```python
from build123d import *

# Parameters (mm, degrees)
ESQUISSE1_R             = 53.5
ESQUISSE1_R_2           = 1
ESQUISSE1_R_3           = 3
BOSS_EXTRU_1_DEPTH      = 1.6
ENL_V_MAT_EXTRU_1_DEPTH = 76.677341391


with BuildPart() as part:
    # Esquisse1 → Boss.-Extru.1 (new body)
    with BuildSketch(Plane.XY):
        Circle(ESQUISSE1_R)
        with Locations((35, 0)):
            Circle(ESQUISSE1_R_2, mode=Mode.SUBTRACT)
        with Locations((17.5, -30.310889132)):
            Circle(ESQUISSE1_R_2, mode=Mode.SUBTRACT)
        with Locations((-17.5, -30.310889132)):
            Circle(ESQUISSE1_R_2, mode=Mode.SUBTRACT)
        with Locations((-35, 0)):
            Circle(ESQUISSE1_R_2, mode=Mode.SUBTRACT)
        with Locations((-17.5, 30.310889132)):
            Circle(ESQUISSE1_R_2, mode=Mode.SUBTRACT)
        with Locations((17.5, 30.310889132)):
            Circle(ESQUISSE1_R_2, mode=Mode.SUBTRACT)
        with Locations((0, -15)):
            Circle(ESQUISSE1_R_3, mode=Mode.SUBTRACT)
        with Locations((12.990381057, -7.5)):
            Circle(ESQUISSE1_R_3, mode=Mode.SUBTRACT)
        with Locations((12.990381057, 7.5)):
            Circle(ESQUISSE1_R_3, mode=Mode.SUBTRACT)
        with Locations((0, 15)):
            Circle(ESQUISSE1_R_3, mode=Mode.SUBTRACT)
        with Locations((-12.990381057, 7.5)):
            Circle(ESQUISSE1_R_3, mode=Mode.SUBTRACT)
    extrude(amount=BOSS_EXTRU_1_DEPTH)

    # Esquisse2 → Enlèv. mat.-Extru.1 (cut, through all)
    with BuildSketch(Plane.XY.offset(1.6)):
        with BuildLine():
            Line((-37.206596087, 38.4437148), (14.689935589, -51.4437148))
            ThreePointArc((14.689935589, -51.4437148), (-46.332359102, -26.75), (-37.206596087, 38.4437148))
        make_face()
    extrude(amount=-ENL_V_MAT_EXTRU_1_DEPTH, mode=Mode.SUBTRACT)


solid = part.part
```
Here's how the part is built. I have some questions about the finished solid (model axes, mm). Round coordinates to 2 decimals unless told otherwise and drop trailing zeros. Write each loop counter-clockwise with the first axis right and the second up, starting at its lowest first coordinate (ties: lowest second). Pieces come first, ordered by that corner, then holes.
Q1. Please list where these lines run through material, in increasing order: probe 1 along X at (y, z) = (30, 0.7); probe 2 along Y at (x, z) = (17.5, 1.3); probe 3 along Y at (x, z) = (0, 1.1).
Q2. If we section it at A-A on y = -7.5: Write out the boundary of the cut face in (x, z), plus the area to 3 significant figures.
Q3. If we section it at D-D on x = 5.5: Write out the boundary of the cut face in (y, z).
Q4. Will these pins go through, and if not, where does the flat tip stop? P1, Ø9.5, axis at x = -12.99, y = 7.5, coming from the -Z side; P2, Ø1.8, axis at x = -17.5, y = 30.31, coming from the -Z side.
Q5. If we section it at B-B on z = 0.8: Give the number of separate pieces and of enclosed holes in the cut face, plus the area to 3 significant figures.
Q6. If we section it at C-C on y = 7.5: Write out the boundary of the cut face in (x, z).
Q7. If we mould it in two halves opening along Y, with no side actions, what happens to faces 1 (the flat face through (-11.62, -5.87, 0.81)), 2 (the flat face through (18, 13, 1.6)), 3 (the cylindrical face through (10.78, -5.47, 0.79))? For each: +Y half, -Y half, draft (parallel to the pull), parting line (faces both ways), or undercut.
Answer below:
1. probe 1: x = -32.33 to -18.45, -16.55 to 16.55, 18.45 to 44.3
1. probe 2: y = -50.56 to -31.31, -29.31 to 29.31, 31.31 to 50.56
1. probe 3: y = -26 to -18, -12 to 12, 18 to 53.5
2. outline: (-10.68, 0) - (9.99, 0) - (9.99, 1.6) - (-10.68, 1.6) - close; (15.99, 0) - (52.97, 0) - (52.97, 1.6) - (15.99, 1.6) - close
2. area: 92.2 mm2
3. outline: (-35.53, 0) - (53.22, 0) - (53.22, 1.6) - (-35.53, 1.6) - close
4. P1: stops at z = 0
4. P2: passes through
5. separate pieces: 1
5. enclosed holes: 9
5. area: 5,720 mm2
6. outline: (-19.34, 0) - (-15.99, 0) - (-15.99, 1.6) - (-19.34, 1.6) - close; (-9.99, 0) - (9.99, 0) - (9.99, 1.6) - (-9.99, 1.6) - close; (15.99, 0) - (52.97, 0) - (52.97, 1.6) - (15.99, 1.6) - close
7. face 1: -Y half
7. face 2: draft
7. face 3: undercut
